Job drawing, mm, ordinate dimensions from the low corner. One solid piece. A direction names the side the tool comes from. Give positions to 0.01 mm unless a question says otherwise; leave off trailing zeros. Order: outer loops, then holes, each group sorted by start corner. A loop starts at its lowest first (then second) coordinate and runs counter-clockwise, first axis right, second up.
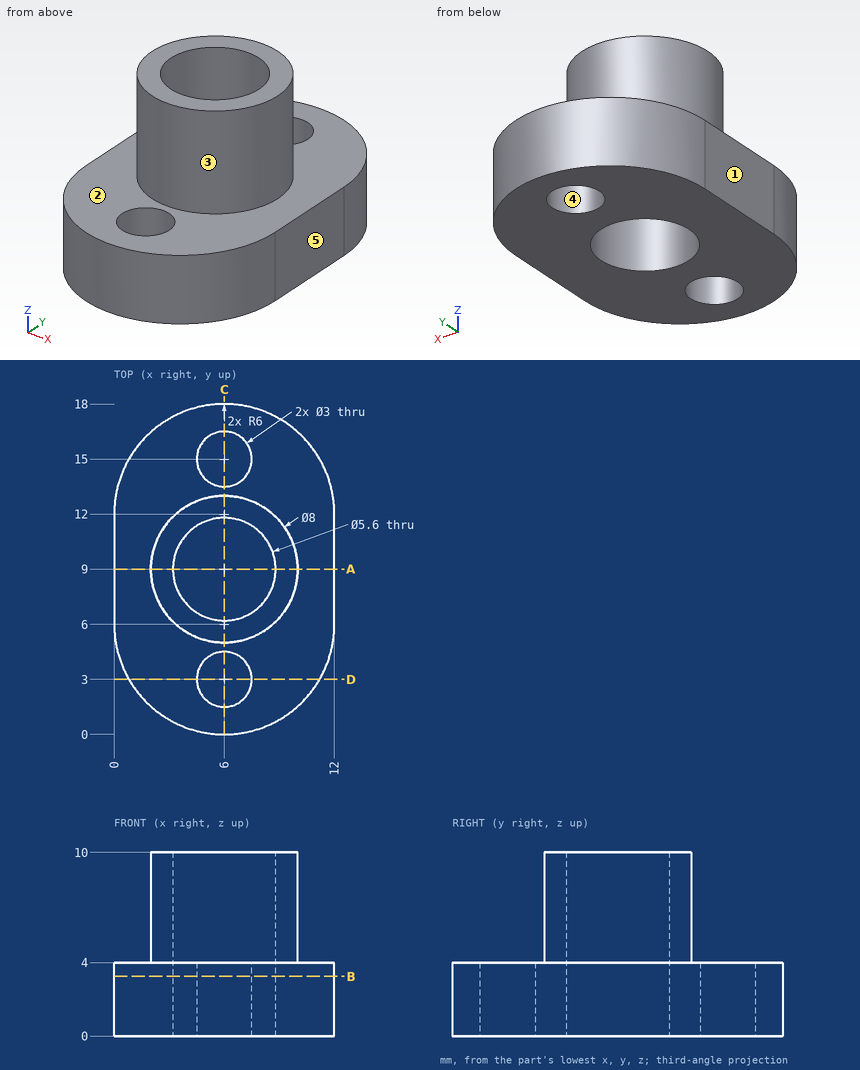
Item 1: Band-saw the part on A-A on y = 9. List the corners of the cut face in (x, z).
Item 2: Pull direction Y, two halves, no side cores. Call the marked faces 3, 4 and 5: released by +Y, released by -Y, zero draft, split by the parting line, or undercut.
Item 3: Band-saw the part on C-C on x = 6. List the corners of the cut face in (y, z), plus the area to 3 significant figures.
Item 4: Band-saw the part on D-D on y = 3. List the corners of the cut face in (x, z), plus the area to 3 significant figures.
Item 5: Drop flat-ended pins along their axis: P1, Ø1.5, axis at y = 5, z = 8.5, coming from the +X side; P2, Ø1.5, axis at x = 4.5, z = 5.5, coming from the +Y side; P3, Ø2, axis at y = 5.5, z = 8.5, coming from the +X side. Give the stop position or say it passes through.
Item 6: Drill centre lines: probe 1 along Y at (x, z) = (6, 3.1); probe 2 along Y at (x, z) = (6, 4.25); probe 3 along Z at (x, y) = (10.25, 13.75). Where is each one in solid material? Low to high.
Item 7: Band-saw the part on B-B on z = 3.25. List the corners of the cut face in (x, y), plus the area to 3 significant figures.
Item 8: Which spindle directions (+Z, -Z, +X, -X, +Y, -Y) get a long thin tool onto all of the face, cutting with end or side? Do the marked faces 1 and 2. Say none if no direction does.
Working result:
1. outline: (0, 0) - (3.2, 0) - (3.2, 10) - (2, 10) - (2, 4) - (0, 4) - close; (8.8, 0) - (12, 0) - (12, 4) - (10, 4) - (10, 10) - (8.8, 10) - close
2. face 3: split by the parting line
2. face 4: undercut
2. face 5: zero draft
3. outline: (0, 0) - (1.5, 0) - (1.5, 4) - (0, 4) - close; (4.5, 0) - (6.2, 0) - (6.2, 10) - (5, 10) - (5, 4) - (4.5, 4) - close; (11.8, 0) - (13.5, 0) - (13.5, 4) - (13, 4) - (13, 10) - (11.8, 10) - close; (16.5, 0) - (18, 0) - (18, 4) - (16.5, 4) - close
3. area: 40.0 mm2
4. outline: (0.8, 0) - (4.5, 0) - (4.5, 4) - (0.8, 4) - close; (7.5, 0) - (11.2, 0) - (11.2, 4) - (7.5, 4) - close
4. area: 29.6 mm2
5. P1: stops at x = 8.33
5. P2: stops at y = 12.93
5. P3: stops at x = 9.12
6. probe 1: y = 0 to 1.5, 4.5 to 6.2, 11.8 to 13.5, 16.5 to 18
6. probe 2: y = 5 to 6.2, 11.8 to 13
6. probe 3: z = 0 to 4
7. outline: (0, 6) arc R6 ccw to (12, 6) - (12, 12) arc R6 ccw to (0, 12) - close; hole circle Ø5.6 at (6, 9); hole circle Ø3 at (6, 3); hole circle Ø3 at (6, 15)
7. area: 146 mm2
8. face 1: +Z, -Z, -X, +Y, -Y
8. face 2: +Z
